Source: CAD feature listing. Evaluate the final solid. Frame: model axes, mm. Face numbers are marked on the shaded views. Round coordinates to 2 decimals unless told otherwise and drop trailing zeros. Loops run counter-clockwise (first coordinate to the right, second up) from the corner with the lowest first, then second, coordinate; pieces in that order, holes last.
(1) Mould query, pull axis X, two halves, no side actions, for the marked faces 1, 2, 3 and 4. Classes: pulls with the +X half, pulls with the -X half, needs draft (parallel to the pull), parting line crosses it, or undercut.
(2) Section C-C, the plane x = -11.5. Return the cut outline in (y, z), plus the area to 3 significant figures.
(3) First-contact query: pin 1 Ø3 at (x, y) = (33.5, -7.5) entering from -Z; pin 2 Ø3 at (x, z) = (26.165, 8) entering from -Y. Flat tips, straight axial feed; report the tip coordinate or a pass-through.
(4) Section A-A, the plane x = 50. Return the cut outline in (y, z), plus the area to 3 significant figures.
(5) Section B-B, the plane y = -9. Return the cut outline in (x, z), plus the area to 3 significant figures.
(6) Material intervals for probe 1 along X at (y, z) = (-9.25, 10.25); probe 2 along Y at (x, z) = (63.9, 8); probe 3 along Z at (x, y) = (61.4, -9), sorted ascending.
```python
from build123d import *

# Parameters (mm, degrees)
EXTRUDE_2_DEPTH          = 16
SKETCH_3_R               = 1.65
CUT_EXTRUDE_1_DEPTH      = 126
CUT_EXTRUDE_1_DEPTH_BACK = 6
EXTRUDE_3_DEPTH          = 3
MIRROR_2_COPY_1_DEPTH    = 3
SKETCH_7_W               = 24
SKETCH_7_H               = 12
CUT_EXTRUDE_2_DEPTH      = 5
SKETCH_10_R              = 1
CUT_EXTRUDE_3_DEPTH      = 5


with BuildPart() as part:
    # 草图1 → 凸台-拉伸2 (new body)
    with BuildSketch(Plane.XY):
        Polygon((-65, 0), (65, 0), (65, -12), (60, -12), (60, -5), (-60, -5), (-60, -12), (-65, -12), align=None)
    extrude(amount=EXTRUDE_2_DEPTH)

    # 草图3 → 切除-拉伸1 (cut, two sides)
    with BuildSketch(Plane(origin=(-60, 0, 0), x_dir=(0, 0, -1), z_dir=(1, 0, 0))) as cut_extrude_1_sk:
        with Locations((-8, -9)):
            Circle(SKETCH_3_R)
    extrude(amount=CUT_EXTRUDE_1_DEPTH, mode=Mode.SUBTRACT)
    extrude(cut_extrude_1_sk.sketch, amount=-CUT_EXTRUDE_1_DEPTH_BACK, mode=Mode.SUBTRACT)

    # 草图4 → 凸台-拉伸3 (add)
    with BuildSketch(Plane(origin=(0, 0, 0), x_dir=(-1, 0, 0), z_dir=(0, 0, -1))):
        Polygon((54, -5), (60, -12), (60, -5), align=None)
    extrude_3 = extrude(amount=-EXTRUDE_3_DEPTH)

    # 镜向1: 凸台-拉伸3 across plane
    add(extrude_3.mirror(Plane.XY.offset(8)))

    # 镜向2: 凸台-拉伸3 across plane
    add(extrude_3.mirror(Plane(origin=(0, 0, 0), x_dir=(0, 0, 1), z_dir=(1, 0, 0))))

    # 镜向2 copy 1 sketch → 镜向2 copy 1 (add)
    with BuildSketch(Plane.XY.offset(16)):
        Polygon((54, -5), (60, -12), (60, -5), align=None)
    extrude(amount=-MIRROR_2_COPY_1_DEPTH)

    # 草图7 → 切除-拉伸2 (cut)
    with BuildSketch(Plane.XZ.offset(5)):
        with Locations((40, 8)):
            Rectangle(SKETCH_7_W, SKETCH_7_H)
    extrude(amount=-CUT_EXTRUDE_2_DEPTH, mode=Mode.SUBTRACT)

    # 草图10 → 切除-拉伸3 (cut)
    with BuildSketch(Plane.XZ.offset(5)):
        with Locations((53.835, 8)):
            Circle(SKETCH_10_R)
        with Locations((26.165, 8)):
            Circle(SKETCH_10_R)
    extrude(amount=-CUT_EXTRUDE_3_DEPTH, mode=Mode.SUBTRACT)


solid = part.part
```
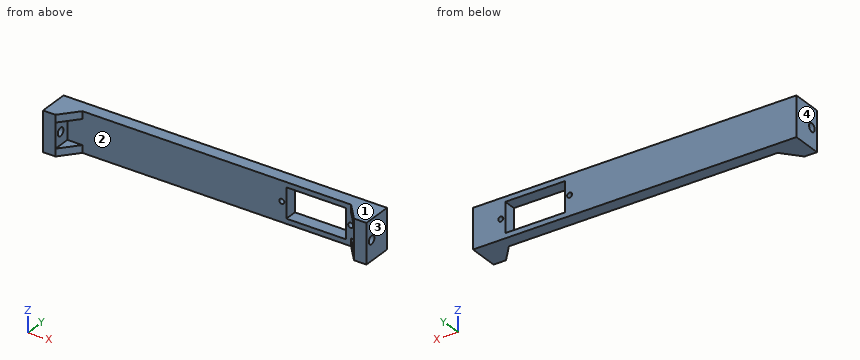
Output values:
1. face 1: needs draft
1. face 2: undercut
1. face 3: pulls with the +X half
1. face 4: pulls with the -X half
2. outline: (-5, 0) - (0, 0) - (0, 16) - (-5, 16) - close
2. area: 80.0 mm2
3. pin 1: passes through
3. pin 2: stops at y = -5
4. outline: (-5, 0) - (0, 0) - (0, 2) - (-5, 2) - close; (-5, 14) - (0, 14) - (0, 16) - (-5, 16) - close
4. area: 20.0 mm2
5. outline: (-65, 0) - (-57.43, 0) - (-57.43, 3) - (-60, 3) - (-60, 6.35) - (-65, 6.35) - close; (-65, 9.65) - (-60, 9.65) - (-60, 13) - (-57.43, 13) - (-57.43, 16) - (-65, 16) - close; (57.43, 0) - (65, 0) - (65, 6.35) - (60, 6.35) - (60, 3) - (57.43, 3) - close; (57.43, 13) - (60, 13) - (60, 9.65) - (65, 9.65) - (65, 16) - (57.43, 16) - close
5. area: 158 mm2
6. probe 1: x = -65 to -60, 60 to 65
6. probe 2: y = -12 to -10.65, -7.35 to 0
6. probe 3: z = 0 to 6.35, 9.65 to 16
